```python
from build123d import *

# Parameters (mm, degrees)
SKETCH_1_W                         = 400
SKETCH_1_H                         = 144
SKETCH_1_R                         = 4.25
SM_BASE_FLANGE_1_DEPTH             = 0.7
SM_EDGE_FLANGE_1_STRIP_W           = 3.2
SM_EDGE_FLANGE_1_STRIP_H           = 0.7
SM_EDGE_FLANGE_1_STRIP_CUT_DEPTH   = 400
SM_EDGE_FLANGE_1_STRIP_2_W         = 3.2
SM_EDGE_FLANGE_1_STRIP_2_H         = 0.7
SM_EDGE_FLANGE_1_STRIP_CUT_2_DEPTH = 400
SM_EDGE_FLANGE_1_DEPTH             = 400
SM_EDGE_FLANGE_1_BEND_DEPTH        = 400
SKETCH_14_R                        = 3
CUT_EXTRUDE_1_DEPTH                = 10
CUT_EXTRUDE_START                  = -10
SKETCH_15_R                        = 3
CUT_EXTRUDE_2_DEPTH                = 10


# Sheet-metal steps are written as plain solids
with BuildPart() as part:
    # Sketch 1 → 基体-法兰1 (new body)
    with BuildSketch(Plane(origin=(0, 0, 0), x_dir=(1, 0, 0), z_dir=(0, 1, 0))):
        Rectangle(SKETCH_1_W, SKETCH_1_H)
        with Locations(Location((-175, -48, 0), (0, 0, 270))):
            Circle(SKETCH_1_R, mode=Mode.SUBTRACT)
        with Locations(Location((-175, -24, 0), (0, 0, 270))):
            Circle(SKETCH_1_R, mode=Mode.SUBTRACT)
        with Locations(Location((-175, 0, 0), (0, 0, 270))):
            Circle(SKETCH_1_R, mode=Mode.SUBTRACT)
        with Locations(Location((-175, 24, 0), (0, 0, 270))):
            Circle(SKETCH_1_R, mode=Mode.SUBTRACT)
        with Locations(Location((-175, 48, 0), (0, 0, 270))):
            Circle(SKETCH_1_R, mode=Mode.SUBTRACT)
        with Locations(Location((-125, -48, 0), (0, 0, 90))):
            Circle(SKETCH_1_R, mode=Mode.SUBTRACT)
        with Locations(Location((-125, -24, 0), (0, 0, 90))):
            Circle(SKETCH_1_R, mode=Mode.SUBTRACT)
        with Locations(Location((-125, 0, 0), (0, 0, 90))):
            Circle(SKETCH_1_R, mode=Mode.SUBTRACT)
        with Locations(Location((-125, 24, 0), (0, 0, 90))):
            Circle(SKETCH_1_R, mode=Mode.SUBTRACT)
        with Locations(Location((-125, 48, 0), (0, 0, 90))):
            Circle(SKETCH_1_R, mode=Mode.SUBTRACT)
        with Locations(Location((-75, -48, 0), (0, 0, 270))):
            Circle(SKETCH_1_R, mode=Mode.SUBTRACT)
        with Locations(Location((-25, -48, 0), (0, 0, 90))):
            Circle(SKETCH_1_R, mode=Mode.SUBTRACT)
        with Locations(Location((-25, -24, 0), (0, 0, 90))):
            Circle(SKETCH_1_R, mode=Mode.SUBTRACT)
        with Locations(Location((-75, -24, 0), (0, 0, 270))):
            Circle(SKETCH_1_R, mode=Mode.SUBTRACT)
        with Locations(Location((-75, 0, 0), (0, 0, 270))):
            Circle(SKETCH_1_R, mode=Mode.SUBTRACT)
        with Locations(Location((-25, 0, 0), (0, 0, 90))):
            Circle(SKETCH_1_R, mode=Mode.SUBTRACT)
        with Locations(Location((-75, 24, 0), (0, 0, 270))):
            Circle(SKETCH_1_R, mode=Mode.SUBTRACT)
        with Locations(Location((-25, 24, 0), (0, 0, 90))):
            Circle(SKETCH_1_R, mode=Mode.SUBTRACT)
        with Locations(Location((-25, 48, 0), (0, 0, 90))):
            Circle(SKETCH_1_R, mode=Mode.SUBTRACT)
        with Locations(Location((-75, 48, 0), (0, 0, 270))):
            Circle(SKETCH_1_R, mode=Mode.SUBTRACT)
        with Locations(Location((25, 48, 0), (0, 0, 270))):
            Circle(SKETCH_1_R, mode=Mode.SUBTRACT)
        with Locations(Location((25, 24, 0), (0, 0, 270))):
            Circle(SKETCH_1_R, mode=Mode.SUBTRACT)
        with Locations(Location((25, 0, 0), (0, 0, 270))):
            Circle(SKETCH_1_R, mode=Mode.SUBTRACT)
        with Locations(Location((25, -24, 0), (0, 0, 270))):
            Circle(SKETCH_1_R, mode=Mode.SUBTRACT)
        with Locations(Location((25, -48, 0), (0, 0, 270))):
            Circle(SKETCH_1_R, mode=Mode.SUBTRACT)
        with Locations(Location((75, -48, 0), (0, 0, 90))):
            Circle(SKETCH_1_R, mode=Mode.SUBTRACT)
        with Locations(Location((75, -24, 0), (0, 0, 90))):
            Circle(SKETCH_1_R, mode=Mode.SUBTRACT)
        with Locations(Location((75, 0, 0), (0, 0, 90))):
            Circle(SKETCH_1_R, mode=Mode.SUBTRACT)
        with Locations(Location((75, 24, 0), (0, 0, 90))):
            Circle(SKETCH_1_R, mode=Mode.SUBTRACT)
        with Locations(Location((75, 48, 0), (0, 0, 90))):
            Circle(SKETCH_1_R, mode=Mode.SUBTRACT)
        with Locations(Location((125, 48, 0), (0, 0, 270))):
            Circle(SKETCH_1_R, mode=Mode.SUBTRACT)
        with Locations(Location((125, 24, 0), (0, 0, 270))):
            Circle(SKETCH_1_R, mode=Mode.SUBTRACT)
        with Locations(Location((125, 0, 0), (0, 0, 270))):
            Circle(SKETCH_1_R, mode=Mode.SUBTRACT)
        with Locations(Location((125, -24, 0), (0, 0, 270))):
            Circle(SKETCH_1_R, mode=Mode.SUBTRACT)
        with Locations(Location((125, -48, 0), (0, 0, 270))):
            Circle(SKETCH_1_R, mode=Mode.SUBTRACT)
        with Locations(Location((175, -48, 0), (0, 0, 90))):
            Circle(SKETCH_1_R, mode=Mode.SUBTRACT)
        with Locations(Location((175, -24, 0), (0, 0, 90))):
            Circle(SKETCH_1_R, mode=Mode.SUBTRACT)
        with Locations(Location((175, 0, 0), (0, 0, 90))):
            Circle(SKETCH_1_R, mode=Mode.SUBTRACT)
        with Locations(Location((175, 24, 0), (0, 0, 90))):
            Circle(SKETCH_1_R, mode=Mode.SUBTRACT)
        with Locations(Location((175, 48, 0), (0, 0, 90))):
            Circle(SKETCH_1_R, mode=Mode.SUBTRACT)
    extrude(amount=-SM_BASE_FLANGE_1_DEPTH)

    # 边线-法兰1 strip (across the edge) → 边线-法兰1 strip cut (cut)
    with BuildSketch(Plane(origin=(-200, 0, 72), x_dir=(0, 0, -1), z_dir=(1, 0, 0))):
        with Locations((-0.7, -0.35)):
            Rectangle(SM_EDGE_FLANGE_1_STRIP_W, SM_EDGE_FLANGE_1_STRIP_H)
    extrude(amount=SM_EDGE_FLANGE_1_STRIP_CUT_DEPTH, mode=Mode.SUBTRACT)

    # 边线-法兰1 strip 2 (across the edge) → 边线-法兰1 strip cut 2 (cut)
    with BuildSketch(Plane(origin=(200, 0, -72), x_dir=(0, 0, 1), z_dir=(-1, 0, 0))):
        with Locations((-0.7, -0.35)):
            Rectangle(SM_EDGE_FLANGE_1_STRIP_2_W, SM_EDGE_FLANGE_1_STRIP_2_H)
    extrude(amount=SM_EDGE_FLANGE_1_STRIP_CUT_2_DEPTH, mode=Mode.SUBTRACT)

    # 边线-法兰1 section (across the edge) → 边线-法兰1 (add)
    with BuildSketch(Plane(origin=(-200, 0, 72), x_dir=(0, 0, -1), z_dir=(1, 0, 0))):
        with BuildLine():
            Line((0, 0.2), (0, 13.3))
            Line((0, 13.3), (0.7, 13.3))
            Line((0.7, 13.3), (0.7, 0.2))
            ThreePointArc((0.7, 0.2), (0.758578644, 0.058578644), (0.9, 0))
            Line((0.9, 0), (0.9, -0.7))
            ThreePointArc((0.9, -0.7), (0.263603897, -0.436396103), (0, 0.2))
        make_face()
    extrude(amount=SM_EDGE_FLANGE_1_DEPTH)

    # 边线-法兰1 section 2 (across the edge) → 边线-法兰1 bend (add)
    with BuildSketch(Plane(origin=(200, 0, -72), x_dir=(0, 0, 1), z_dir=(-1, 0, 0))):
        with BuildLine():
            Line((0, 0.2), (0, 13.3))
            Line((0, 13.3), (0.7, 13.3))
            Line((0.7, 13.3), (0.7, 0.2))
            ThreePointArc((0.7, 0.2), (0.758578644, 0.058578644), (0.9, 0))
            Line((0.9, 0), (0.9, -0.7))
            ThreePointArc((0.9, -0.7), (0.263603897, -0.436396103), (0, 0.2))
        make_face()
    extrude(amount=SM_EDGE_FLANGE_1_BEND_DEPTH)

    # 草图14 → 切除-拉伸1 (cut)
    with BuildSketch(Plane.XY.offset(72)):
        with Locations((-194.5, 7.8)):
            Circle(SKETCH_14_R)
        with Locations((0, 7.8)):
            Circle(SKETCH_14_R)
        with Locations(Location((194.5, 7.8, 0), (0, 0, 180))):
            Circle(SKETCH_14_R)
    extrude(amount=-CUT_EXTRUDE_1_DEPTH, mode=Mode.SUBTRACT)

    # 草图15 → 切除-拉伸2 (cut)
    with BuildSketch(Plane(origin=(0, 0, -72), x_dir=(-1, 0, 0), z_dir=(0, 0, -1)).offset(CUT_EXTRUDE_START)):
        with Locations((-194.5, 7.8)):
            Circle(SKETCH_15_R)
        with Locations(Location((0, 7.8, 0), (0, 0, 180))):
            Circle(SKETCH_15_R)
        with Locations(Location((194.5, 7.8, 0), (0, 0, 180))):
            Circle(SKETCH_15_R)
    extrude(amount=CUT_EXTRUDE_2_DEPTH, mode=Mode.SUBTRACT)


solid = part.part
```
Source: CAD feature listing. Evaluate the final solid. Frame: model axes, mm. Round coordinates to 2 decimals unless told otherwise and drop trailing zeros. Order: outer loops, then holes, each group sorted by start corner. A loop starts at its lowest first (then second) coordinate and runs counter-clockwise, first axis right, second up. Notation, with made-up numbers: (64.5, 89.25) -> (99.5, 89.25) arc R13 cw to (99.5, 102.25) -> close; hole circle Ø2 at (45.5, -18.5). An arc over 180 degrees is marked (long way). One line per item, written item: value. Start each with the question number.
Q1. Draft query along Z for faces 1 (the flat face through (3, 5, -72)), 2 (the cylindrical face through (78.77, -0.35, -25.96)), 3 (the flat face through (-3, -0.7, -1)). Return one class per face: pulls with the +Z half, pulls with the -Z half, needs draft (parallel to the pull), parting line crosses it, or undercut.
Q2. Pin query (flat end, axial travel): pin 1 (11 mm diameter, centred on x = -75, z = -48, fed in from +Y). Return the tip coordinate at first contact, or that it passes through.
Q3. Section query A-A (x = -125). Give the number of separate pieces and of enclosed holes in the cut face, plus the area to 3 significant figures.
Q4. Section query C-C (x = 104). Return the cut outline in (y, z), plus the area to 3 significant figures.
Q5. Section query D-D (z = 35). Return the cut outline in (x, y).
Q6. Material intervals for probe 1 along Z at (x, y) = (96, 4.75); probe 2 along Z at (x, y) = (-25, -0.15); probe 3 along Y at (x, z) = (-82, -42.5), sorted ascending.
Findings below:
1. face 1: pulls with the -Z half
1. face 2: undercut
1. face 3: needs draft
2. pin 1: y = 0
3. separate pieces: 6
3. enclosed holes: 0
3. area: 89.3 mm²
4. outline: (-0.7, -71.1) arc R0.9 ccw to (0.2, -72) -> (13.3, -72) -> (13.3, -71.3) -> (0.2, -71.3) arc R0.2 cw to (0, -71.1) -> (0, 71.1) arc R0.2 cw to (0.2, 71.3) -> (13.3, 71.3) -> (13.3, 72) -> (0.2, 72) arc R0.9 ccw to (-0.7, 71.1) -> close
4. area: 119 mm²
5. outline: (-200, -0.7) -> (200, -0.7) -> (200, 0) -> (-200, 0) -> close
6. probe 1: -72 to -71.3, 71.3 to 72
6. probe 2: -71.93 to -52.25, -43.75 to -28.25, -19.75 to -4.25, 4.25 to 19.75, 28.25 to 43.75, 52.25 to 71.93
6. probe 3: -0.7 to 0
